The model under review builds one solid part; all positions refer to its coordinate system, in mm. Face numbers are marked on the shaded views. A direction names the side the tool comes from. Give positions to 0.01 mm unless a question says otherwise; leave off trailing zeros. Write each loop counter-clockwise with the first axis right and the second up, starting at its lowest first coordinate (ties: lowest second). Pieces come first, ordered by that corner, then holes. Notation, with made-up numbers: (53.5, 60.5) - (86.5, 60.5) arc R26 cw to (86.5, 74.5) - close; hole circle Ø4 at (49, 10.5). An arc over 180 degrees is marked (long way). Write item = value, one per line.
```python
from build123d import *

# Parameters (mm, degrees)
SKETCH003_R  = 7.46
PAD002_DEPTH = 25
SKETCH006_R  = 6
PAD005_DEPTH = 60
SKETCH007_R  = 1.5
PAD006_DEPTH = 10
SKETCH008_R  = 3
PAD007_DEPTH = 3
SKETCH_W     = 60
SKETCH_H     = 105
SKETCH_W_2   = 43
SKETCH_H_2   = 60
PAD_DEPTH    = 5
SKETCH005_W  = 8
SKETCH005_H  = 10
SKETCH005_R  = 2
PAD004_DEPTH = 8.5
SKETCH004_W  = 8
SKETCH004_H  = 10
SKETCH004_R  = 2
PAD003_DEPTH = 8.5
PAD001_DEPTH = 5
CHAMFER_SIZE = 15


with BuildPart() as bearingslot:
    # Sketch003 → Pad002 (new body)
    with BuildSketch(Plane.YZ.offset(17.5)):
        with Locations((10, 10)):
            Circle(SKETCH003_R)
        with Locations((95, 10)):
            Circle(SKETCH003_R)
    extrude(amount=PAD002_DEPTH)


with BuildPart() as rodslot:
    # Sketch006 → Pad005 (new body)
    with BuildSketch(Plane.YZ):
        with Locations((10, 10)):
            Circle(SKETCH006_R)
        with Locations((95, 10)):
            Circle(SKETCH006_R)
    extrude(amount=PAD005_DEPTH)


with BuildPart() as mountpoints:
    # Sketch007 → Pad006 (new body)
    with BuildSketch(Plane.XY.offset(10)):
        with Locations((4, 19.25)):
            Circle(SKETCH007_R)
        with Locations((56, 19.25)):
            Circle(SKETCH007_R)
        with Locations((56, 85.75)):
            Circle(SKETCH007_R)
        with Locations((4, 85.75)):
            Circle(SKETCH007_R)
    extrude(amount=-PAD006_DEPTH)


with BuildPart() as cutblocks:
    # Sketch008 → Pad007 (new body)
    with BuildSketch(Plane.XY):
        with Locations((4, 85.75)):
            Circle(SKETCH008_R)
        with Locations((56, 85.75)):
            Circle(SKETCH008_R)
        with Locations((56, 19.25)):
            Circle(SKETCH008_R)
        with Locations((4, 19.25)):
            Circle(SKETCH008_R)
    extrude(amount=PAD007_DEPTH)

    # Fusion: union BearingSlot, RodSlot, MountPoints
    add(bearingslot.part)
    add(rodslot.part)
    add(mountpoints.part)


with BuildPart() as base:
    # Sketch → Pad (new body)
    with BuildSketch(Plane.XY):
        with Locations((30, 52.5)):
            Rectangle(SKETCH_W, SKETCH_H)
        with Locations((30, 52.5)):
            Rectangle(SKETCH_W_2, SKETCH_H_2, mode=Mode.SUBTRACT)
    extrude(amount=PAD_DEPTH)


with BuildPart() as obj1:
    # Sketch005 → Pad004 (new body)
    with BuildSketch(Plane.YZ.offset(60)):
        with Locations((78.5, 10)):
            Rectangle(SKETCH005_W, SKETCH005_H)
        with Locations((78.5, 11)):
            Circle(SKETCH005_R, mode=Mode.SUBTRACT)
    extrude(amount=-PAD004_DEPTH)


with BuildPart() as obj2:
    # Sketch004 → Pad003 (new body)
    with BuildSketch(Plane.YZ):
        with Locations((78.5, 10)):
            Rectangle(SKETCH004_W, SKETCH004_H)
        with Locations((78.5, 11)):
            Circle(SKETCH004_R, mode=Mode.SUBTRACT)
    extrude(amount=PAD003_DEPTH)


with BuildPart() as chamfer_body:
    # Pad001 base: copy of Base
    add(base.part)

    # Sketch001 → Pad001 (new body)
    with BuildSketch(Plane.XY.offset(5)):
        Polygon((16.5, 105), (43.5, 105), (43.5, 92.5), (60, 92.5), (60, 82.5), (0, 82.5), (0, 92.5), (16.5, 92.5), align=None)
        Polygon((0, 22.5), (60, 22.5), (60, 12.5), (43.5, 12.5), (43.5, 0), (16.5, 0), (16.5, 12.5), (0, 12.5), align=None)
    extrude(amount=PAD001_DEPTH)

    # Fusion001: union Base, obj1, obj2
    add(base.part)
    add(obj1.part)
    add(obj2.part)

    # Cut: cut CutBlocks
    add(cutblocks.part, mode=Mode.SUBTRACT)

    # Chamfer
    chamfer_edges = [chamfer_body.edges().sort_by_distance(p)[0] for p in [
        (0, 105, 2.5),
        (60, 0, 2.5),
        (60, 105, 2.5),
        (0, 0, 2.5),
    ]]
    chamfer(chamfer_edges, length=CHAMFER_SIZE)


solid = chamfer_body.part
```
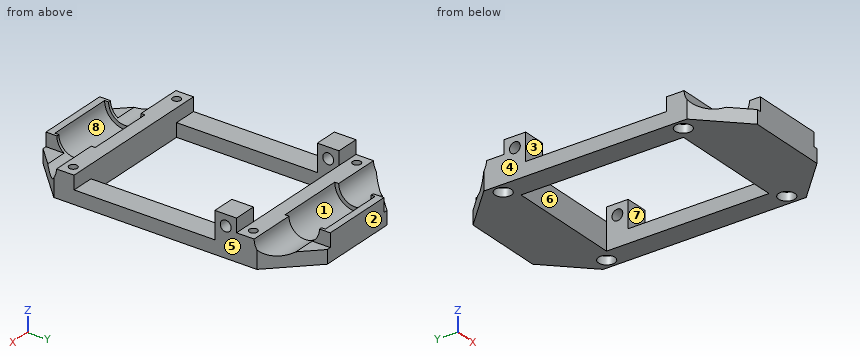
1. Take a section at B-B on y = 78.5. Give the boundary of the cut face in (x, z), and give its area (3 significant figures).
Findings below:
outline = (0, 0) - (8.5, 0) - (8.5, 9) - (0, 9) - close; (0, 13) - (8.5, 13) - (8.5, 15) - (0, 15) - close; (51.5, 0) - (60, 0) - (60, 9) - (51.5, 9) - close; (51.5, 13) - (60, 13) - (60, 15) - (51.5, 15) - close
area = 187 mm²
2. Take a section at D-D on x = 56. Count the separate pieces of the cut face and the enclosed holes in it, and give its area (3 significant figures).
Findings below:
separate_pieces = 3
enclosed_holes = 1
area = 475 mm²
3. Draft analysis for pull direction Y (two halves, no side actions). For the marked faces 1, 2, 3 and 4, state which applies: +Y half, -Y half, draft (parallel to the pull), parting line (faces both ways), or undercut.
Findings below:
face_1 = undercut
face_2 = +Y half
face_3 = undercut
face_4 = draft
4. For line 1 (Y direction, x = 16, z = 3); line 2 (X direction, y = 85.5, z = 7.75); line 3 (Y direction, x = 4, z = 5.25), list the stretches that pass through material, from the lowest coordinate up. Write a range as from..to.
Findings below:
line_1 = 0..22.5, 82.5..105
line_2 = 0..2.52, 5.48..54.52, 57.48..60
line_3 = 13.67..17.75, 20.75..22.5, 74.5..84.25, 87.25..91.33
5. Take a section at A-A on x = 14. Give the boundary of the cut face in (y, z).
Findings below:
outline = (1, 0) - (22.5, 0) - (22.5, 10) - (16, 10) arc R6 cw to (6.68, 5) - (1, 5) - close; (82.5, 0) - (104, 0) - (104, 5) - (98.32, 5) arc R6 cw to (89, 10) - (82.5, 10) - close
6. Take a section at C-C on y = 38.5. Give the boundary of the cut face in (x, z).
Findings below:
outline = (0, 0) - (8.5, 0) - (8.5, 5) - (0, 5) - close; (51.5, 0) - (60, 0) - (60, 5) - (51.5, 5) - close
7. Machinability: for the marked faces 5, 6, 7 and 8, which of the approach directions +Z, -Z, +X, -X, +Y, -Y give a long, thin tool a straight path to every point of the face, cutting with its end or side? Answer none if there is none.
Findings below:
face_5 = +Z, -Z, +X, +Y, -Y
face_6 = +Z, -Z
face_7 = +Z, +X, -X
face_8 = +Z
8. Insertion check: P1, Ø2, axis at x = 11, z = 10.5, coming from the -Y side; P2, Ø2.5, axis at x = 57.5, y = 38, coming from the +Z side; P3, Ø1.8, axis at x = 55, y = 85.5, coming from the -Z side; P4, Ø1.8, axis at x = 56, y = 85.75, coming from the -Z side. Each pin has a flat end and moves straight along its axis. Give the tip position at first contact, or say it passes through.
Findings below:
P1 = 15.98
P2 = 5
P3 = 3
P4 = through
